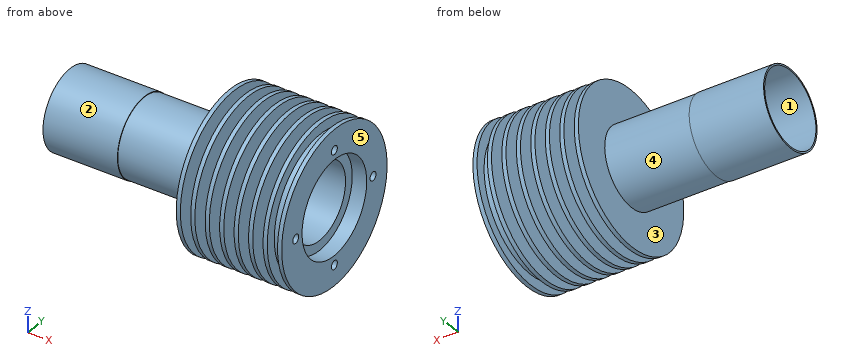
from build123d import *

# Parameters (mm, degrees)
SKETCH1_W                 = 36
SKETCH1_H                 = 0.75
M5X0_8_TAPPED_HOLE3_D     = 4.2
M5X0_8_TAPPED_HOLE3_DEPTH = 9


with BuildPart() as part:
    # Sketch1 → Revolve1 (revolve)
    with BuildSketch(Plane.XY, mode=Mode.PRIVATE) as revolve1_sk:
        with Locations((-110, 18.625)):
            Rectangle(SKETCH1_W, SKETCH1_H)
        Polygon((-92, 18.75), (-92, 18.25), (-9, 18.25), (-9, 18.75), (-14, 18.75), (-14, 37.5), (-16, 37.5), (-16, 18.75), (-21, 18.75), (-21, 37.5), (-23, 37.5), (-23, 18.75), (-28, 18.75), (-28, 37.5), (-30, 37.5), (-30, 18.75), (-35, 18.75), (-35, 37.5), (-37, 37.5), (-37, 18.75), (-42, 18.75), (-42, 37.5), (-44, 37.5), (-44, 18.75), (-49, 18.75), (-49, 37.5), (-51, 37.5), (-51, 18.75), (-56, 18.75), align=None)
        Polygon((-7, 18.25), (-9, 18.25), (-9, 37.5), (-7, 37.5), (-7, 32.5), (-2, 32.5), (-2, 37.5), (0, 37.5), (0, 23), (-7, 23), align=None)
    revolve(revolve1_sk.sketch.rotate(Axis((0, 0, 0), (-1, 0, 0)), 90), axis=Axis((0, 0, 0), (-1, 0, 0)))

    # M5x0.8 Tapped Hole3
    with Locations(Plane(origin=(0, 0, 0), x_dir=(0, 0, -1), z_dir=(1, 0, 0))):
        with Locations((0, 27.5), (-27.5, 0), (0, -27.5), (27.5, 0)):
            Hole(M5X0_8_TAPPED_HOLE3_D / 2, depth=M5X0_8_TAPPED_HOLE3_DEPTH)


solid = part.part
Build history of the part. All positions in model axes, mm. Face numbers are marked on the shaded views. A direction names the side the tool comes from. Coordinates: 2 decimals unless noted, no trailing zeros. Write each loop counter-clockwise with the first axis right and the second up, starting at its lowest first coordinate (ties: lowest second). Pieces come first, ordered by that corner, then holes. Notation, with made-up numbers: (81, 74) -> (104, 74) arc R31 cw to (104, 111) -> close; hole circle Ø5 at (8.25, 81). An arc over 180 degrees is marked (long way). Use CSV: the item, a comma, the result in double quotes. Start each with the question number.
Q1. Cut at B-B, the plane y = 0. State how many separate pieces and enclosed holes the cut face has, then the cut area to 3 significant figures.
Q2. Pull direction Y, two halves, no side cores. Call the marked faces 1, 2 and 3: released by +Y, released by -Y, zero draft, split by the parting line, or undercut.
Q3. 3-axis set-ups, long thin cutter, end or side, ignore diameter. For the marked faces 4 and 5: which of +Z, -Z, +X, -X, +Y, -Y reach the whole face in a straight line?
Q4. Cut at A-A, the plane x = -114. List the corners of the cut face in (y, z).
Q5. Cut at D-D, the plane x = -87. List the corners of the cut face in (y, z), then the cut area to 3 significant figures.
Q6. Drill centre lines: probe 1 along Y at (x, z) = (-70, 0); probe 2 along Z at (x, y) = (-34, -16); probe 3 along Z at (x, y) = (-32, -13). Where is each one in solid material? Low to high.
Q7. Flat gauge pins, fed straight in: pin 1 Ø8 at (x, z) = (-103, -8) entering from -Y; pin 2 Ø1 at (x, y) = (-67.5, 4.5) entering from -Z; pin 3 Ø5 at (x, z) = (-16.5, 29.5) entering from +Y. Where does each tip first touch, or does it go through?
Checked values:
1,separate pieces,"4"
1,enclosed holes,"0"
1,area,"741 mm²"
2,face 1,"undercut"
2,face 2,"split by the parting line"
2,face 3,"zero draft"
3,face 4,"none"
3,face 5,"+Z, -Z, +X, +Y, -Y"
4,outline,"circle Ø38 at (0, 0); hole circle Ø36.5 at (0, 0)"
5,outline,"circle Ø37.5 at (0, 0); hole circle Ø36.5 at (0, 0)"
5,area,"58.1 mm²"
6,probe 1,"y = -18.75 to -18.25, 18.25 to 18.75"
6,probe 2,"z = -9.78 to -8.78, 8.78 to 9.78"
6,probe 3,"z = -13.51 to -12.81, 12.81 to 13.51"
7,pin 1,"stops at y = -18.57"
7,pin 2,"stops at z = -18.32"
7,pin 3,"stops at y = 25.97"
